Autodesk Inventor part; units mm, degrees
ref_plane "YZ Plane" through (0, 0, 0) normal (1, 0, 0) x (0, 1, 0)
ref_plane "XZ Plane" through (0, 0, 0) normal (0, 1, 0) x (-1, 0, 0)
ref_plane "XY Plane" through (0, 0, 0) normal (0, 0, 1) x (1, 0, 0)
sketch "Sketch1" plane through (0, 0, 0) normal (0, 0, 1) x (1, 0, 0)
  circle A0 centre (0, 0) radius 20.5 construction
  line L0 (0, 0) -> (29, 0)
  circle A1 centre (24.75, 0) radius 4.25
  circle A2 centre (24.75, 0) radius 3 construction
  circle A3 centre (24.75, 0) radius 3.05 construction
  circle A4 centre (24.75, 0) radius 2.75 construction
  circle A5 centre (24.75, 0) radius 3.25 construction
  circle A6 centre (0, 0) radius 22.5
  circle A7 centre (12.375, 21.4341) radius 4.25
  circle A8 centre (-12.375, 21.4341) radius 4.25
  circle A9 centre (-24.75, 0) radius 4.25
  circle A10 centre (-12.375, -21.4341) radius 4.25
  circle A11 centre (12.375, -21.4341) radius 4.25
  point P0 (22.2374, -3.4277)
  point P1 (22.2374, 3.4277)
  point P2 (14.5, 25.1147)
  point P3 (-14.5, 25.1147)
  point P4 (-29, 0)
  point P5 (-14.5, -25.1147)
  point P6 (14.5, -25.1147)
  point P7 (14.0872, 17.5443)
  point P8 (8.1502, 20.972)
  point P9 (-8.1502, 20.972)
  point P10 (-14.0872, 17.5443)
  point P11 (-22.2374, -3.4277)
  point P12 (-22.2374, 3.4277)
  point P13 (-14.0872, -17.5443)
  point P14 (-8.1502, -20.972)
  point P15 (8.1502, -20.972)
  point P16 (14.0872, -17.5443)
  dimension "InsideDiameter" = 41
  dimension "SpacerOuterDiameter" = 6
  dimension "SpacerGap" = 0.05
  dimension "M3_HeadDiameter" = 5.5
  dimension "HeadDiameterThickness" = 0.5
  dimension "WallThickness" = 1
  dimension "d38" = 2
  dimension "d41" = 360
extrude "Extrusion1" add sketch "Sketch1" against normal blind 5
hole "Hole1" at (0, 0, 0) direction (0, 0, -1) diameter 37.5 end through all counterbore diameter 41 counterbore depth 2.5
hole "Hole2" at (24.75, 0, 0) at (12.375, -21.4341, 0) at (-12.375, -21.4341, 0) at (-12.375, 21.4341, 0) at (12.375, 21.4341, 0) direction (0, 0, -1) diameter 3.5 end through all counterbore diameter 6.1 counterbore depth 3.5
hole "Hole3" at (-24.75, 0, 0) direction (0, 0, -1) diameter 3.5 end through all counterbore diameter 6.1 counterbore depth 1.5
fillet "Fillet1" radius 2 12 edges at (22.2374, 3.4277, -2.5) (22.2374, -3.4277, -2.5) (14.0872, -17.5443, -2.5) (8.1502, -20.972, -2.5) (-14.0872, -17.5443, -2.5) (-8.1502, -20.972, -2.5) (-22.2374, -3.4277, -2.5) (-22.2374, 3.4277, -2.5) (-14.0872, 17.5443, -2.5) (-8.1502, 20.972, -2.5) (8.1502, 20.972, -2.5) (14.0872, 17.5443, -2.5)
equation "\"InsideDiameter_\" = InsideDiameter"
equation "\"SpacerDiameter\" = SpacerOuterDiameter + 2 * SpacerGap"
equation "\"d33\" = SpacerOuterDiameter + 2 * SpacerGap"
properties part number "CrossRollerBearingOuterSupportStand" material "Aluminum 7075"
Geometry: final body of the model. Coordinates: model frame, mm. A direction names the side the tool comes from. Coordinates: 2 decimals unless noted, no trailing zeros. Loops run counter-clockwise (first coordinate to the right, second up) from the corner with the lowest first, then second, coordinate; pieces in that order, holes last. Notation, with made-up numbers: (-7.75, -28) - (44.25, -28) arc R30 ccw to (44.25, 8) - close; hole circle Ø7 at (56, 4). An arc over 180 degrees is marked (long way). Put each result on its own line as item: value. Start each with the question number.
Q1. Cut plane C-C, the plane y = 8. Return loops of the section in (x, z), and give its area (3 significant figures).
Q2. Cut plane A-A, the plane x = -24.75. Return loops of the section in (y, z), and give its area (3 significant figures).
Q3. Line query: line 1 (Y direction, x = 24.5, z = -1.85); line 2 (Y direction, x = -14, z = -1.55); line 3 (X direction, y = -0.5, z = -4.6). Output: solid intervals per line, ascending.
Q4. Set-up query: faces 1 (the cylindrical face through (-26.485, 0.228, -3.274)), 2 (the cylindrical face through (22.69, 2.25, -1.77)). Return all of +Z, -Z, +X, -X, +Y, -Y with unobstructed straight access to the full face (end or side cutting, diameter ignored); none if empty.
Q5. Pull-direction query (X, two-part tool) for faces 3 (the cylindrical face through (-19.528, -11.176, -2.465)), 4 (the flat face through (-15.2, -11.3, -5)), 5 (the flat face through (-23, -1, -1.5)); classes: released by +X, released by -X, zero draft, split by the parting line, or undercut.
Q6. Cut plane D-D, the plane x = 19.5. Return loops of the section in (y, z).
Q7. Pin query (flat end, axial travel): pin 1 Ø3 at (x, y) = (11.5, -21) entering from +Z; pin 2 Ø3 at (x, z) = (-2, -3) entering from -Y; pin 3 Ø1 at (y, z) = (-3.5, -2.5) entering from -X; pin 4 Ø3 at (x, y) = (-24.75, 0) entering from -Z. Return the tip coordinate at first contact, or that it passes through.
Q8. Cut plane B-B, the plane y = 0. Return loops of the section in (x, z).
Filled sheet:
1. outline: (-21.03, -5) - (-16.96, -5) - (-16.96, -2.5) - (-18.87, -2.5) - (-18.87, 0) - (-21.03, 0) - close; (16.96, -5) - (21.03, -5) - (21.03, 0) - (18.87, 0) - (18.87, -2.5) - (16.96, -2.5) - close
1. area: 31.1 mm²
2. outline: (-4.25, -5) - (-1.75, -5) - (-1.75, -1.5) - (-3.05, -1.5) - (-3.05, 0) - (-4.25, 0) - close; (1.75, -5) - (4.25, -5) - (4.25, 0) - (3.05, 0) - (3.05, -1.5) - (1.75, -1.5) - close
2. area: 21.1 mm²
3. line 1: -4.24 to -3.04, 3.04 to 4.24
3. line 2: -25.36 to -24.02, -18.85 to -14.97, 14.97 to 18.85, 24.02 to 25.36
3. line 3: -28.97 to -26.43, -23.07 to -18.74, 18.74 to 23.07, 26.43 to 28.97
4. face 1: +Z, -Z
4. face 2: +Z
5. face 3: released by -X
5. face 4: zero draft
5. face 5: undercut
6. outline: (-11.22, -5) - (11.22, -5) - (11.22, 0) - (6.32, 0) - (6.32, -2.5) - (-6.32, -2.5) - (-6.32, 0) - (-11.22, 0) - close
7. pin 1: z = -3.5
7. pin 2: y = -22.49
7. pin 3: x = -27.76
7. pin 4: through
8. outline: (-29, -5) - (-26.5, -5) - (-26.5, -1.5) - (-27.8, -1.5) - (-27.8, 0) - (-29, 0) - close; (-23, -5) - (-18.75, -5) - (-18.75, -2.5) - (-20.5, -2.5) - (-20.5, 0) - (-21.7, 0) - (-21.7, -1.5) - (-23, -1.5) - close; (18.75, -5) - (23, -5) - (23, -3.5) - (21.7, -3.5) - (21.7, 0) - (20.5, 0) - (20.5, -2.5) - (18.75, -2.5) - close; (26.5, -5) - (29, -5) - (29, 0) - (27.8, 0) - (27.8, -3.5) - (26.5, -3.5) - close
